```python
from build123d import *

# Parameters (mm, degrees)
ESQUISSE1_W        = 13
ESQUISSE1_H        = 9.5
BOSS_EXTRU_1_DEPTH = 8
ESQUISSE2_R        = 4
BOSS_EXTRU_2_DEPTH = 1
ESQUISSE3_R        = 3
BOSS_EXTRU_3_DEPTH = 9
ESQUISSE4_W        = 2
ESQUISSE4_H        = 0.8
BOSS_EXTRU_4_DEPTH = 4


with BuildPart() as part:
    # Esquisse1 → Boss.-Extru.1 (new body)
    with BuildSketch(Plane(origin=(0, 0, 0), x_dir=(0, 0, -1), z_dir=(1, 0, 0))):
        with Locations((6.5, 4.75)):
            Rectangle(ESQUISSE1_W, ESQUISSE1_H)
    extrude(amount=BOSS_EXTRU_1_DEPTH)

    # Esquisse2 → Boss.-Extru.2 (add)
    with BuildSketch(Plane(origin=(0, 9.5, 0), x_dir=(1, 0, 0), z_dir=(0, 1, 0))):
        with Locations((4, 6.5)):
            Circle(ESQUISSE2_R)
    extrude(amount=BOSS_EXTRU_2_DEPTH)

    # Esquisse3 → Boss.-Extru.3 (add)
    with BuildSketch(Plane(origin=(0, 10.5, 0), x_dir=(1, 0, 0), z_dir=(0, 1, 0))):
        with Locations((4, 6.5)):
            Circle(ESQUISSE3_R)
    extrude(amount=BOSS_EXTRU_3_DEPTH)

    # Esquisse4 → Boss.-Extru.4 (add)
    with BuildSketch(Plane.XZ):
        with Locations((4, -3)):
            Rectangle(ESQUISSE4_W, ESQUISSE4_H)
        with Locations((4, -6.5)):
            Rectangle(ESQUISSE4_W, ESQUISSE4_H)
        with Locations((4, -10)):
            Rectangle(ESQUISSE4_W, ESQUISSE4_H)
    extrude(amount=BOSS_EXTRU_4_DEPTH)


solid = part.part
```
Here's how the part is built. I have some questions about the finished solid (model axes, mm). A direction names the side the tool comes from. Coordinates: 2 decimals unless noted, no trailing zeros. Loops run counter-clockwise (first coordinate to the right, second up) from the corner with the lowest first, then second, coordinate; pieces in that order, holes last. Notation, with made-up numbers: (63, -20.5) - (71, -20.5) arc R20 cw to (71, -5.5) - close; hole circle Ø5 at (52.5, -23). An arc over 180 degrees is marked (long way). Return JSON: item names as keys, results as strings. Group by question number.
Item 1: We'd pull the mould along Z, two halves only. Please class faces 1 (the face through (4, -2, -9.6)), 2 (the face through (1, 10.5, -8)), 3 (the face through (4, -2, -2.6)): +Z half, -Z half, draft (parallel to the pull), parting line (faces both ways), or undercut.
Item 2: If we section it at C-C on y = 14.75: Write out the boundary of the cut face in (x, z).
Item 3: Will these pins go through, and if not, where does the flat tip stop? P1, Ø2, axis at x = 4, y = -1.5, coming from the -Z side; P2, Ø1.5, axis at y = 12, z = -8, coming from the -X side; P3, Ø1, axis at x = 3.5, y = -1.5, coming from the +Z side.
Item 4: If we section it at A-A on x = 4: Write out the boundary of the cut face in (y, z), and give its area (3 significant figures).
Item 5: If we section it at D-D on x = 2.5: Write out the boundary of the cut face in (y, z).
Item 6: If we section it at B-B on z = -11.5: Write out the boundary of the cut face in (x, y).
Item 7: I need wall thicknesses on line 1 (Y direction, x = 5.5, z = -7.5); line 2 (Y direction, x = 0.5, z = -3); line 3 (Z direction, x = 6.5, y = 11.5). Which ranges of each line are inside material? Lowest first, please. Write a range as from..to.
Item 8: On a 3-axis mill with a long thin cutter (end or side, diameter ignored), from which of +Z, -Z, +X, -X, +Y, -Y can I reach the whole of each face in a straight line? I mean faces 4 (the face through (4, -2, -3.4)), 5 (the face through (3, -2, -6.5)), 6 (the face through (5, -2, -10)), 7 (the face through (4, -2, -10.4)), 8 (the face through (4, 9.5, -11)). Say none if no direction works.
Calculated:
{
 "1": {"face 1": "undercut", "face 2": "draft", "face 3": "+Z half"},
 "2": {"outline": "circle Ø6 at (4, -6.5)"},
 "3": {"P1": "stops at z = -10.4", "P2": "stops at x = 1.1", "P3": "stops at z = -2.6"},
 "4": {"outline": "(-4, -10.4) - (0, -10.4) - (0, -13) - (9.5, -13) - (9.5, -10.5) - (10.5, -10.5) - (10.5, -9.5) - (19.5, -9.5) - (19.5, -3.5) - (10.5, -3.5) - (10.5, -2.5) - (9.5, -2.5) - (9.5, 0) - (0, 0) - (0, -2.6) - (-4, -2.6) - (-4, -3.4) - (0, -3.4) - (0, -6.1) - (-4, -6.1) - (-4, -6.9) - (0, -6.9) - (0, -9.6) - (-4, -9.6) - close", "area": "195 mm^2"},
 "5": {"outline": "(0, -13) - (9.5, -13) - (9.5, -10.21) - (10.5, -10.21) - (10.5, -9.1) - (19.5, -9.1) - (19.5, -3.9) - (10.5, -3.9) - (10.5, -2.79) - (9.5, -2.79) - (9.5, 0) - (0, 0) - close"},
 "6": {"outline": "(0, 0) - (8, 0) - (8, 9.5) - (0, 9.5) - close"},
 "7": {"line 1": "y = 0..19.5", "line 2": "y = 0..9.5", "line 3": "z = -8.16..-4.84"},
 "8": {"face 4": "+X, -X, -Y", "face 5": "+Z, -Z, -X, -Y", "face 6": "+Z, -Z, +X, -Y", "face 7": "-Z, +X, -X, -Y", "face 8": "-Z, +Y"}
}
